```python
from build123d import *

# Parameters (mm, degrees)
SKETCH7_W           = 4.7625
SKETCH7_H           = 2.12122512
BOSS_EXTRUDE2_DEPTH = 47.09795
SKETCH8_W           = 2.12122512
SKETCH8_H           = 4.7625
BOSS_EXTRUDE3_DEPTH = 47.09795
BOSS_EXTRUDE4_DEPTH = 47.09795


with BuildPart() as part:
    # Sketch7 → Boss-Extrude2 (new, symmetric)
    with BuildSketch(Plane.XY):
        with Locations((-4.92125, -2.560612608)):
            Rectangle(SKETCH7_W, SKETCH7_H)
    extrude(amount=BOSS_EXTRUDE2_DEPTH, both=True)



with BuildPart() as body_2:
    # Sketch8 → Boss-Extrude3 (new, symmetric)
    with BuildSketch(Plane.XY):
        with Locations((2.560612608, 4.92125)):
            Rectangle(SKETCH8_W, SKETCH8_H)
    extrude(amount=BOSS_EXTRUDE3_DEPTH, both=True)


with BuildPart() as part_1:
    add(part.part)

    add(body_2.part)  # Boss-Extrude4 merges body 2
    # Sketch11 → Boss-Extrude4 (add, symmetric)
    with BuildSketch(Plane.XY):
        with BuildLine():
            Line((-2.54, -1.500000048), (-7.3025, -1.500000048))
            Line((-7.3025, -1.500000048), (-7.3025, -3.621225168))
            Line((-7.3025, -3.621225168), (-2.54, -3.621225168))
            ThreePointArc((-2.54, -3.621225168), (1.816644097, -1.816644097), (3.621225168, 2.54))
            Line((3.621225168, 2.54), (3.621225168, 7.3025))
            Line((3.621225168, 7.3025), (1.500000048, 7.3025))
            Line((1.500000048, 7.3025), (1.500000048, 2.54))
            Line((1.500000048, 2.54), (-1.500000048, 2.54))
            ThreePointArc((-1.500000048, 2.54), (-1.804608982, 1.804608982), (-2.54, 1.500000048))
            Line((-2.54, 1.500000048), (-2.54, -1.500000048))
        make_face()
    extrude(amount=BOSS_EXTRUDE4_DEPTH, both=True)


solid = part_1.part
```
Work out the finished part from the listing and answer in its coordinate system (mm). A direction names the side the tool comes from. Give positions to 0.01 mm unless a question says otherwise; leave off trailing zeros. Write each loop counter-clockwise with the first axis right and the second up, starting at its lowest first coordinate (ties: lowest second). Pieces come first, ordered by that corner, then holes. Notation, with made-up numbers: (-32.5, 16.25) - (-8.5, 16.25) arc R24 ccw to (-8.5, 27.25) - close; hole circle Ø4 at (73, 11). An arc over 180 degrees is marked (long way). Use one line per item in the form item = value.
1. Each of these flat-tipped pins is pushed along its axis until it touches: pin 1 Ø1 at (y, z) = (-0.5, 12) entering from +X; pin 2 Ø2.5 at (x, z) = (0, -2.5) entering from +Y; pin 3 Ø4 at (x, z) = (0.5, -12) entering from -Y. Where does it stop, or does it pass through?
Filled in:
pin_1 = 3.07
pin_2 = 2.54
pin_3 = -3.53
2. For faces 4 (the face through (3, 7.302, 1)), 5 (the face through (-5, -1.5, 1)), determine the directions among +Z, -Z, +X, -X, +Y, -Y from which every point of the face is accessible in a straight line to the end or side of a thin tool.
Filled in:
face_4 = +Z, -Z, +X, -X, +Y
face_5 = +Z, -Z, -X, +Y
3. Determine the mould class of faces 1 (the face through (-1, 1, -47.098)), 2 (the face through (-1, 1, 47.098)), 3 (the face through (-2.54, 0, 1)) for opening direction Z: released by +Z, released by -Z, zero draft, split by the parting line, or undercut.
Filled in:
face_1 = released by -Z
face_2 = released by +Z
face_3 = zero draft
4. A cutting plane is placed at B-B (y = 6.5). Write down the section's boundary in (x, z).
Filled in:
outline = (1.5, -47.1) - (3.62, -47.1) - (3.62, 47.1) - (1.5, 47.1) - close
5. Consider L1, parallel to X at y = 6.75, z = 6.5; L2, parallel to Y at x = -4, z = -19; L3, parallel to Y at x = -2.5, z = -42.5. Determine where each line is inside the solid, lowest interval first.
Filled in:
L1 = 1.5 to 3.62
L2 = -3.62 to -1.5
L3 = -3.62 to 1.5
6. A cutting plane is placed at A-A (z = 15.5). Write down the section's boundary in (x, y), and give its area (3 significant figures).
Filled in:
outline = (-7.3, -3.62) - (-2.54, -3.62) arc R6.16 ccw to (3.62, 2.54) - (3.62, 7.3) - (1.5, 7.3) - (1.5, 2.54) - (-1.5, 2.54) arc R1.04 cw to (-2.54, 1.5) - (-2.54, -1.5) - (-7.3, -1.5) - close
area = 49.2 mm^2
7. A cutting plane is placed at C-C (x = -5.5). Write down the section's boundary in (y, z), and give its area (3 significant figures).
Filled in:
outline = (-3.62, -47.1) - (-1.5, -47.1) - (-1.5, 47.1) - (-3.62, 47.1) - close
area = 200 mm^2
